Source: CAD feature listing. Evaluate the final solid. Frame: model axes, mm. Face numbers are marked on the shaded views. Give positions to 0.01 mm unless a question says otherwise; leave off trailing zeros. Order: outer loops, then holes, each group sorted by start corner. A loop starts at its lowest first (then second) coordinate and runs counter-clockwise, first axis right, second up.
from build123d import *
from OCP.BRepFilletAPI import BRepFilletAPI_MakeChamfer

# Parameters (mm, degrees)
SKETCH1_R           = 57.5
BOSS_EXTRUDE1_DEPTH = 600
SKETCH2_R           = 43.291669187
CUT_EXTRUDE1_DEPTH  = 606.485342515
CHAMFER1_SIZE       = 7.78529
CHAMFER1_SIZE2      = 4.494839


with BuildPart() as part:
    # Sketch1 → Boss-Extrude1 (new body)
    with BuildSketch(Plane(origin=(0, 0, 0), x_dir=(1, 0, 0), z_dir=(0, 1, 0))):
        with Locations(Location((0, 0, 0), (0, 0, 270))):
            Circle(SKETCH1_R)
    extrude(amount=BOSS_EXTRUDE1_DEPTH)

    # Sketch2 → Cut-Extrude1 (cut, through all)
    with BuildSketch(Plane(origin=(0, 0, 0), x_dir=(1, 0, 0), z_dir=(0, 1, 0))):
        with Locations(Location((0, 0, 0), (0, 0, 270))):
            Circle(SKETCH2_R)
    extrude(amount=CUT_EXTRUDE1_DEPTH, mode=Mode.SUBTRACT)

    # Chamfer1: one chamfer whose edges measure the first distance from different faces: ONE call of the kernel's chamfer builder (chamfer() names one face for all edges)
    chamfer1_edges_1 = [part.edges().sort_by_distance(p)[0] for p in [
        (0, 0, -57.5),
    ]]
    chamfer1_side_1 = [part.faces().sort_by_distance(p)[0] for p in [
        (0, 300, -57.5),
    ]]
    chamfer1_edges_2 = [part.edges().sort_by_distance(p)[0] for p in [
        (0, 600, -57.5),
    ]]
    chamfer1_side_2 = [part.faces().sort_by_distance(p)[0] for p in [
        (0, 600, -55.873654403),
    ]]
    chamfer1 = BRepFilletAPI_MakeChamfer(part.part.solid().wrapped)
    for e in chamfer1_edges_1:
        chamfer1.Add(CHAMFER1_SIZE, CHAMFER1_SIZE2, e.wrapped, chamfer1_side_1[0].wrapped)  # the first distance lies on this face
    for e in chamfer1_edges_2:
        chamfer1.Add(CHAMFER1_SIZE, CHAMFER1_SIZE2, e.wrapped, chamfer1_side_2[0].wrapped)  # the first distance lies on this face
    add(Compound.cast(chamfer1.Shape()), mode=Mode.REPLACE)


solid = part.part
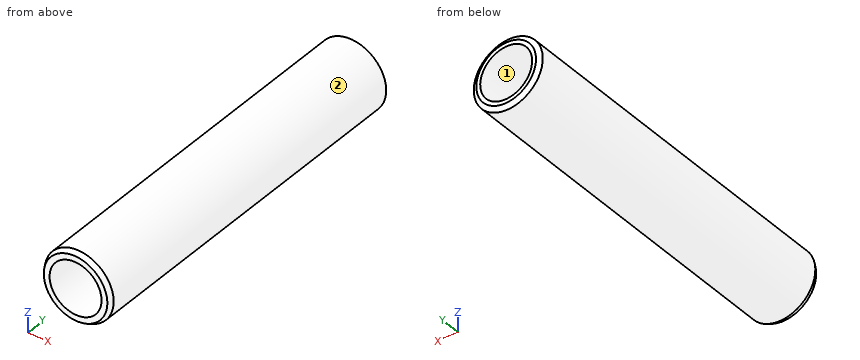
1) Section query A-A on z = 0. Output: boundary loops of the cut face in (x, y), and give its area (3 significant figures).
Checks:
outline: (-57.5, 7.79) - (-53.01, 0) - (-43.29, 0) - (-43.29, 600) - (-49.71, 600) - (-57.5, 595.51) - close; (43.29, 0) - (53.01, 0) - (57.5, 7.79) - (57.5, 595.51) - (49.71, 600) - (43.29, 600) - close
area: 17,000 mm2
2) Pull-direction query (X, two-part tool) for the marked faces 1 and 2; classes: +X half, -X half, draft (parallel to the pull), parting line (faces both ways), or undercut.
Checks:
face 1: undercut
face 2: parting line
3) Ray query, L1, parallel to X at y = 146, z = 0; L2, parallel to Z at x = 2.5, y = 292.5; L3, parallel to X at y = 329, z = -12. Return the intervals inside material, ascending.
Checks:
L1: x = -57.5 to -43.29, 43.29 to 57.5
L2: z = -57.45 to -43.22, 43.22 to 57.45
L3: x = -56.23 to -41.6, 41.6 to 56.23
4) Section query C-C on y = 485. Output: boundary loops of the cut face in (x, z), and give its area (3 significant figures).
Checks:
outline: circle Ø115 at (0, 0); hole circle Ø86.58 at (0, 0)
area: 4,500 mm2
5) Section query B-B on x = 0. Output: boundary loops of the cut face in (y, z).
Checks:
outline: (0, -53.01) - (7.79, -57.5) - (595.51, -57.5) - (600, -49.71) - (600, -43.29) - (0, -43.29) - close; (0, 43.29) - (600, 43.29) - (600, 49.71) - (595.51, 57.5) - (7.79, 57.5) - (0, 53.01) - close
6) First-contact query: pin 1 Ø4 at (x, y) = (-24, 508.5) entering from +Z; pin 2 Ø5 at (y, z) = (134.5, -30.5) entering from -X; pin 3 Ø5 at (y, z) = (285.5, -28) entering from -X. Flat tips, straight axial feed; report the tip coordinate or a pass-through.
Checks:
pin 1: stops at z = 53.12
pin 2: stops at x = -50.22
pin 3: stops at x = -51.54
